from build123d import *

# Parameters (mm, degrees)
F1_DEPTH    = 50
F2_W        = 48
F2_H        = 0.5
F2_H_2      = 1.5
F3_DEPTH    = 50
F4_T1_DEPTH = 65.1327459504


# Not quite as in the source:
# - a fillet or chamfer that OpenCascade refuses, or shapes differently, is made with other operations: its cross-section is extruded or revolved along the edge and cut away or added


with BuildPart() as f1:
    # F0 (on Front) → F1 (new body)
    with BuildSketch(Plane.XZ):
        with BuildLine():
            Line((25, -25), (25, 25))
            Line((25, 25), (-25, 25))
            Line((-25, 25), (-25, -25))
            ThreePointArc((-25, -25), (0, -20), (25, -25))
        make_face()
        with BuildLine():
            Line((-20, 20), (20, 20))
            Line((20, 20), (20, -20))
            ThreePointArc((20, -20), (0, -16.5685424949), (-20, -20))
            Line((-20, -20), (-20, 20))
        make_face(mode=Mode.SUBTRACT)
    extrude(amount=F1_DEPTH)

    # F2 (on face) → F3 (cut)
    with BuildSketch(Plane.XZ.offset(50)):
        with Locations((0, 24.75)):
            Rectangle(F2_W, F2_H)
        with Locations((0, 25.75)):
            Rectangle(F2_W, F2_H_2)
        with BuildLine():
            Line((-24, -24.0930467578), (-24, -24.5930467578))
            ThreePointArc((-24, -24.5930467578), (0, -20), (24, -24.5930467578))
            Line((24, -24.5930467578), (24, -24.0930467578))
            ThreePointArc((24, -24.0930467578), (0, -19.5376937746), (-24, -24.0930467578))
        make_face()
    extrude(amount=-F3_DEPTH, mode=Mode.SUBTRACT)

    # F4: fillet of radius 5.08 on 2 edges, made by hand

    # F4_s2 → F4_t1 (cut)
    with BuildSketch(Plane.XZ.offset(-7.5663729752)):
        with BuildLine():
            ThreePointArc((25, 21.9734508099), (24.7435256815, 23.567188555), (24, 25))
            Line((24, 25), (25, 25))
            Line((25, 25), (25, 21.9734508099))
        make_face()
        with BuildLine():
            ThreePointArc((-25, 21.9734508099), (-24.7435256815, 23.567188555), (-24, 25))
            Line((-24, 25), (-25, 25))
            Line((-25, 25), (-25, 21.9734508099))
        make_face()
    extrude(amount=F4_T1_DEPTH, mode=Mode.SUBTRACT)


solid = f1.part
Read the model definition and answer for the solid it produces. Units are mm, in the model's axes. A direction names the side the tool comes from. Give positions to 0.01 mm unless a question says otherwise; leave off trailing zeros. Write each loop counter-clockwise with the first axis right and the second up, starting at its lowest first coordinate (ties: lowest second). Pieces come first, ordered by that corner, then holes. Notation, with made-up numbers: (37, -35.5) - (78, -35.5) arc R34 cw to (78, 2.5) - close; hole circle Ø5 at (41.25, 61.25). An arc over 180 degrees is marked (long way). Use CSV: the item, a comma, the result in double quotes. Start each with the question number.
Item 1: Flat-ended cylindrical pins translate along their axes: P1, Ø4, axis at x = 17.5, z = 16.5, coming from the +Y side; P2, Ø10, axis at x = -7, y = -31, coming from the +Z side; P3, Ø0.6, axis at y = -18, z = 24.5, coming from the -X side; P4, Ø0.6, axis at y = -36.5, z = 25, coming from the +X side. Find the tip coordinate at first contact, or state that the pin passes through.
Item 2: Consider line 1 (X direction, y = -24, z = 3); line 2 (Z direction, x = -6.5, y = -38.5); line 3 (Z direction, x = 3, y = -8.5). Determine where each line is inside the solid, lowest interval first.
Item 3: For faces 1 (the flat face through (0, -25, 24.5)), 2 (the flat face through (0, -25, 20)), 3 (the flat face through (25, -25, -2)), determine the directions among +Z, -Z, +X, -X, +Y, -Y from which every point of the face is accessible in a straight line to the end or side of a thin tool.
Item 4: The mould has two halves that part along X. Classify faces 4 (the cylindrical face through (24.75, -24.65, 23.55)), 5 (the flat face through (20, -25, 0)), 6 (the flat face through (-2, 0, 20.5)): pulls with the +X half, pulls with the -X half, needs draft (parallel to the pull), parting line crosses it, or undercut.
Item 5: The part is cut by section B-B, the plane x = -15. Give the vertices of the cut face in (y, z).
Item 6: The part is cut by section A-A, the plane z = 12.5. Give the vertices of the cut face in (x, y), and give its area (3 significant figures).
Item 7: The part is cut by section C-C, the plane y = -25.5. Give the vertices of the cut face in (x, z), and give its area (3 significant figures).
Taken from the geometry:
1,P1,"through"
1,P2,"z = 24.5"
1,P3,"x = -24.49"
1,P4,"x = 24.21"
2,line 1,"-25 to -20, 20 to 25"
2,line 2,"-19.86 to -16.92, 20 to 24.5"
2,line 3,"-19.61 to -16.64, 20 to 24.5"
3,face 1,"+Z, +Y, -Y"
3,face 2,"+Y, -Y"
3,face 3,"+Z, -Z, +X, +Y, -Y"
4,face 4,"pulls with the +X half"
4,face 5,"undercut"
4,face 6,"needs draft"
5,outline,"(-50, -21.28) - (0, -21.28) - (0, -18.47) - (-50, -18.47) - close; (-50, 20) - (0, 20) - (0, 24.5) - (-50, 24.5) - close"
6,outline,"(-25, -50) - (-20, -50) - (-20, 0) - (-25, 0) - close; (20, -50) - (25, -50) - (25, 0) - (20, 0) - close"
6,area,"500 mm2"
7,outline,"(-25, -25) arc R65 cw to (-24, -24.59) - (-24, -24.09) arc R65.5 cw to (24, -24.09) - (24, -24.59) arc R65 cw to (25, -25) - (25, 21.97) arc R5.08 ccw to (24, 25) - (24, 24.5) - (-24, 24.5) - (-24, 25) arc R5.08 ccw to (-25, 21.97) - close; hole (-20, -20) arc R60 cw to (20, -20) - (20, 20) - (-20, 20) - close"
7,area,"775 mm2"
